from build123d import *

# Parameters (mm, degrees)
BOSS_EXTRUDE1_DEPTH = 6.35
CUT_EXTRUDE1_REACH  = 8.35
SKETCH4_R           = 2.5527
SKETCH4_R_2         = 5.1562
FILLET1_R           = 6.35


with BuildPart() as part:
    # Sketch3 → Boss-Extrude1 (new body)
    with BuildSketch(Plane(origin=(0, 0, 0), x_dir=(1, 0, 0), z_dir=(0, 1, 0))):
        Polygon((0, 0), (191.77, 0), (191.77, -76.2), (152.4, -76.2), (152.4, -39.37), (0, -39.37), align=None)
    extrude(amount=BOSS_EXTRUDE1_DEPTH)

    # Sketch4 → Cut-Extrude1 (cut, up to next)
    with BuildSketch(Plane(origin=(0, 6.35, 0), x_dir=(1, 0, 0), z_dir=(0, 1, 0)), mode=Mode.PRIVATE) as cut_extrude1_sk1:
        with Locations((17.4625, -19.685)):
            Circle(SKETCH4_R)
    cut_extrude1_tool1 = extrude(cut_extrude1_sk1.sketch, amount=-CUT_EXTRUDE1_REACH, mode=Mode.PRIVATE) & part.part
    add(cut_extrude1_tool1.solids().sort_by_distance((17.4625, 6.35, 19.685))[0], mode=Mode.SUBTRACT)
    # Sketch4 → Cut-Extrude1 (cut, up to next)
    with BuildSketch(Plane(origin=(0, 6.35, 0), x_dir=(1, 0, 0), z_dir=(0, 1, 0)), mode=Mode.PRIVATE) as cut_extrude1_sk2:
        with Locations((42.8625, -19.685)):
            Circle(SKETCH4_R)
    cut_extrude1_tool2 = extrude(cut_extrude1_sk2.sketch, amount=-CUT_EXTRUDE1_REACH, mode=Mode.PRIVATE) & part.part
    add(cut_extrude1_tool2.solids().sort_by_distance((42.8625, 6.35, 19.685))[0], mode=Mode.SUBTRACT)
    # Sketch4 → Cut-Extrude1 (cut, up to next)
    with BuildSketch(Plane(origin=(0, 6.35, 0), x_dir=(1, 0, 0), z_dir=(0, 1, 0)), mode=Mode.PRIVATE) as cut_extrude1_sk3:
        with Locations((172.085, -14.2875)):
            Circle(SKETCH4_R_2)
    cut_extrude1_tool3 = extrude(cut_extrude1_sk3.sketch, amount=-CUT_EXTRUDE1_REACH, mode=Mode.PRIVATE) & part.part
    add(cut_extrude1_tool3.solids().sort_by_distance((172.085, 6.35, 14.2875))[0], mode=Mode.SUBTRACT)
    # Sketch4 → Cut-Extrude1 (cut, up to next)
    with BuildSketch(Plane(origin=(0, 6.35, 0), x_dir=(1, 0, 0), z_dir=(0, 1, 0)), mode=Mode.PRIVATE) as cut_extrude1_sk4:
        with Locations((172.085, -61.9125)):
            Circle(SKETCH4_R_2)
    cut_extrude1_tool4 = extrude(cut_extrude1_sk4.sketch, amount=-CUT_EXTRUDE1_REACH, mode=Mode.PRIVATE) & part.part
    add(cut_extrude1_tool4.solids().sort_by_distance((172.085, 6.35, 61.9125))[0], mode=Mode.SUBTRACT)

    # Fillet1
    fillet1_edges = [part.edges().sort_by_distance(p)[0] for p in [
        (0, 3.175, 0),
        (191.77, 3.175, 76.2),
        (152.4, 3.175, 76.2),
        (0, 3.175, 39.37),
    ]]
    fillet(fillet1_edges, radius=FILLET1_R)


solid = part.part
CAD build for the part. Positions are in the model's coordinates, mm. A direction names the side the tool comes from. Round coordinates to 2 decimals unless told otherwise and drop trailing zeros. Order: outer loops, then holes, each group sorted by start corner. A loop starts at its lowest first (then second) coordinate and runs counter-clockwise, first axis right, second up. Notation, with made-up numbers: M -2.5,54 L 24.5,54 A9 cw 24.5,71 Z; hole C 81,51.25 d1. An arc over 180 degrees is marked long. Use one line per item in the form item = value.
Q1. Saw through at A-A on x = 170.5. Give the cut face in (y, z), then the cut area to 3 significant figures.
Recorded:
outline = M 0,0 L 6.35,0 L 6.35,9.38 L 0,9.38 Z; M 0,19.19 L 6.35,19.19 L 6.35,57.01 L 0,57.01 Z; M 0,66.82 L 6.35,66.82 L 6.35,76.2 L 0,76.2 Z
area = 359 mm^2
Q2. Saw through at D-D on z = 53. Give the cut face in (x, y), then the cut area to 3 significant figures.
Recorded:
outline = M 152.4,0 L 191.77,0 L 191.77,6.35 L 152.4,6.35 Z
area = 250 mm^2
Q3. Two-plate mould, pull along Z, no slides. Class faces 3 (the flat face through (0, 3, 20)), 4 (the flat face through (172, 3, 76.2)), 5 (the cylindrical face through (45.297, 3.219, 18.918)): +Z half, -Z half, draft (parallel to the pull), parting line (faces both ways), or undercut.
Recorded:
face_3 = draft
face_4 = +Z half
face_5 = undercut
Q4. Which spindle directions (+Z, -Z, +X, -X, +Y, -Y) get a long thin tool onto all of the face, cutting with end or side? Do faces 1 (the flat face through (98, 3, 0)), 2 (the flat face through (80, 3, 39.37)). Say none if no direction does.
Recorded:
face_1 = -Z, +X, -X, +Y, -Y
face_2 = +Z, -X, +Y, -Y
Q5. Probe L1, parallel to X at y = 4.75, z = 20; L2, parallel to Z at x = 173, y = 4.5; L3, parallel to Z at x = 134, y = 4.75. List the from-to ranges inside material, lowest first.
Recorded:
L1 = 0 to 14.93, 20 to 40.33, 45.4 to 191.77
L2 = 0 to 9.21, 19.36 to 56.84, 66.99 to 76.2
L3 = 0 to 39.37
Q6. Saw through at B-B on y = 4. State how many separate pieces and enclosed holes the cut face has, then the cut area to 3 significant figures.
Recorded:
separate_pieces = 1
enclosed_holes = 4
area = 8,760 mm^2
Q7. Saw through at C-C on x = 136.5. Give the cut face in (y, z), then the cut area to 3 significant figures.
Recorded:
outline = M 0,0 L 6.35,0 L 6.35,39.37 L 0,39.37 Z
area = 250 mm^2
Q8. Flat gauge pins, fed straight in: P1, Ø1.9, axis at x = 96, y = 3, coming from the +Z side; P2, Ø1, axis at y = 4.5, z = 59.5, coming from the -X side. Where does each tip first touch, or does it go through?
Recorded:
P1 = 39.37
P2 = 152.4
